from build123d import *

# Parameters (mm, degrees)
SKETCH1_R           = 40
BOSS_EXTRUDE1_DEPTH = 30
CUT_EXTRUDE1_DEPTH  = 30
SKETCH3_R           = 30
CUT_EXTRUDE2_DEPTH  = 27
SKETCH4_R           = 1.5
SKETCH4_R_2         = 3.5
CUT_EXTRUDE3_DEPTH  = 27


with BuildPart() as part:
    # Sketch1 → Boss-Extrude1 (new body)
    with BuildSketch(Plane.XY):
        Circle(SKETCH1_R)
    extrude(amount=BOSS_EXTRUDE1_DEPTH)

    # Sketch2 → Cut-Extrude1 (cut)
    with BuildSketch(Plane.XY.offset(30)):
        Polygon((4, 40), (-4, 40), (-1.113248654, 35), (1.113248654, 35), align=None)
        Polygon((11.87435719, 32.942965317), (16.16490584, 36.806192674), (8.55645371, 39.278328629), (9.756832416, 33.630990823), align=None)
        Polygon((21.47312091, 27.661243662), (26.747478069, 30.009538766), (20.275342114, 34.711820784), (19.67184675, 28.969945944), align=None)
        Polygon((28.969945944, 19.67184675), (34.711820784, 20.275342114), (30.009538766, 26.747478069), (27.661243662, 21.47312091), align=None)
        Polygon((33.630990823, 9.756832416), (39.278328629, 8.55645371), (36.806192674, 16.16490584), (32.942965317, 11.87435719), align=None)
        Polygon((35, -1.113248654), (40, -4), (40, 4), (35, 1.113248654), align=None)
        Polygon((32.942965317, -11.87435719), (36.806192674, -16.16490584), (39.278328629, -8.55645371), (33.630990823, -9.756832416), align=None)
        Polygon((27.661243662, -21.47312091), (30.009538766, -26.747478069), (34.711820784, -20.275342114), (28.969945944, -19.67184675), align=None)
        Polygon((19.67184675, -28.969945944), (20.275342114, -34.711820784), (26.747478069, -30.009538766), (21.47312091, -27.661243662), align=None)
        Polygon((9.756832416, -33.630990823), (8.55645371, -39.278328629), (16.16490584, -36.806192674), (11.87435719, -32.942965317), align=None)
        Polygon((-1.113248654, -35), (-4, -40), (4, -40), (1.113248654, -35), align=None)
        Polygon((-11.87435719, -32.942965317), (-16.16490584, -36.806192674), (-8.55645371, -39.278328629), (-9.756832416, -33.630990823), align=None)
        Polygon((-21.47312091, -27.661243662), (-26.747478069, -30.009538766), (-20.275342114, -34.711820784), (-19.67184675, -28.969945944), align=None)
        Polygon((-28.969945944, -19.67184675), (-34.711820784, -20.275342114), (-30.009538766, -26.747478069), (-27.661243662, -21.47312091), align=None)
        Polygon((-33.630990823, -9.756832416), (-39.278328629, -8.55645371), (-36.806192674, -16.16490584), (-32.942965317, -11.87435719), align=None)
        Polygon((-35, 1.113248654), (-40, 4), (-40, -4), (-35, -1.113248654), align=None)
        Polygon((-32.942965317, 11.87435719), (-36.806192674, 16.16490584), (-39.278328629, 8.55645371), (-33.630990823, 9.756832416), align=None)
        Polygon((-27.661243662, 21.47312091), (-30.009538766, 26.747478069), (-34.711820784, 20.275342114), (-28.969945944, 19.67184675), align=None)
        Polygon((-19.67184675, 28.969945944), (-20.275342114, 34.711820784), (-26.747478069, 30.009538766), (-21.47312091, 27.661243662), align=None)
        Polygon((-9.756832416, 33.630990823), (-8.55645371, 39.278328629), (-16.16490584, 36.806192674), (-11.87435719, 32.942965317), align=None)
    extrude(amount=-CUT_EXTRUDE1_DEPTH, mode=Mode.SUBTRACT)

    # Sketch3 → Cut-Extrude2 (cut)
    with BuildSketch(Plane.XY.offset(30)):
        Circle(SKETCH3_R)
    extrude(amount=-CUT_EXTRUDE2_DEPTH, mode=Mode.SUBTRACT)

    # Sketch4 → Cut-Extrude3 (cut)
    with BuildSketch(Plane.XY.offset(3)):
        with Locations((8.5, 0)):
            Circle(SKETCH4_R)
        with Locations((-8.5, 0)):
            Circle(SKETCH4_R)
        with Locations((0, -8.5)):
            Circle(SKETCH4_R)
        with Locations((0, 8.5)):
            Circle(SKETCH4_R)
        Circle(SKETCH4_R_2)
    extrude(amount=-CUT_EXTRUDE3_DEPTH, mode=Mode.SUBTRACT)


solid = part.part
The listing builds one solid part. Answer for the finished solid, in the listing's coordinates (mm). A direction names the side the tool comes from. Round coordinates to 2 decimals unless told otherwise and drop trailing zeros. Write each loop counter-clockwise with the first axis right and the second up, starting at its lowest first coordinate (ties: lowest second). Pieces come first, ordered by that corner, then holes. Notation, with made-up numbers: M 7.25,74 L 42.25,74 A22 cw 42.25,107 Z; hole C -39.75,-15 d8. An arc over 180 degrees is marked long. Write each question's results on one line, items separated by ' | '. Start each with the question number.
(1) Find the intervals of material crossed by line 1 (Y direction, x = 0, z = 1.8); line 2 (Y direction, x = 0, z = 20.75); line 3 (Z direction, x = -17, y = 1), in increasing order.
(2) The part is cut by section B-B, the plane y = 13.5. Write down the section's boundary in (x, z), and give its area (3 significant figures).
(3) Determine the mould class of faces 4 (the cylindrical face through (35.655, 18.13, 14.79)), 5 (the flat face through (-24.05, 28.81, 15.21)), 6 (the flat face through (-2.5, 37.4, 15.2)), 7 (the flat face through (-36.31, -9.187, 15.21)) for opening direction X: +X half, -X half, draft (parallel to the pull), parting line (faces both ways), or undercut.
(4) For faces 1 (the flat face through (20.585, -28.306, 15.21)), 2 (the flat face through (37.4, 2.5, 15.2)), 3 (the flat face through (24.05, -28.81, 15.21)), determine the directions among +Z, -Z, +X, -X, +Y, -Y from which every point of the face is accessible in a straight line to the end or side of a thin tool.
(5) The part is cut by section A-A, the plane x = 0. Write down the section's boundary in (y, z), and give its area (3 significant figures).
(6) Each of these flat-tipped pins is pushed along its axis until it touches: P1, Ø1, axis at x = 26.5, z = 5, coming from the -Y side; P2, Ø1.8, axis at y = 0.5, z = 13.5, coming from the +X side; P3, Ø6, axis at y = -30.5, z = 17.5, coming from the +X side. Where does it stop, or does it pass through?
Worked answers:
1) line 1: y = -35 to -10, -7 to -3.5, 3.5 to 7, 10 to 35 | line 2: y = -35 to -30, 30 to 35 | line 3: z = 0 to 3
2) outline: M -34.41,0 L 34.41,0 L 34.41,30 L 26.79,30 L 26.79,3 L -26.79,3 L -26.79,30 L -34.41,30 Z | area: 618 mm²
3) face 4: +X half | face 5: undercut | face 6: undercut | face 7: -X half
4) face 1: +Z, -Z | face 2: +Z, -Z, +X | face 3: +Z, -Z, -Y
5) outline: M -35,0 L -10,0 L -10,3 L -30,3 L -30,30 L -35,30 Z; M -7,0 L -3.5,0 L -3.5,3 L -7,3 Z; M 3.5,0 L 7,0 L 7,3 L 3.5,3 Z; M 10,0 L 35,0 L 35,30 L 30,30 L 30,3 L 10,3 Z | area: 441 mm²
6) P1: stops at y = -29.92 | P2: stops at x = 35.5 | P3: stops at x = 29.05
